Geometry: final body of the model. Coordinates: model frame, mm. Face numbers are marked on the shaded views. A direction names the side the tool comes from. Give positions to 0.01 mm unless a question says otherwise; leave off trailing zeros. Write each loop counter-clockwise with the first axis right and the second up, starting at its lowest first coordinate (ties: lowest second). Pieces come first, ordered by that corner, then holes. Notation, with made-up numbers: (-22, -0.75) -> (22, -0.75) arc R23 ccw to (22, 13.25) -> close; hole circle Ø9 at (16.25, -4.75). An arc over 180 degrees is marked (long way). Answer in a Markdown table with one row per item. Add a question column.
Item 1: Section query B-B on y = 51. Output: boundary loops of the cut face in (x, z) (3 decimals), plus the area to 3 significant figures.
Item 2: Section query A-A on z = -3.5. Output: boundary loops of the cut face in (x, y) (3 decimals).
Item 3: Draft query along X for the marked faces 4, 5, 6 and 7. Return one class per face: +X half, -X half, draft (parallel to the pull), parting line (faces both ways), or undercut.
Item 4: Access query for the marked faces 1, 2 and 3. Directions: +Z, -Z, +X, -X, +Y, -Y. A direction counts if a zero-diameter tool reaches every point of the face in a straight line with its end or side. Return the directions, or none.
Item 5: Material intervals for probe 1 along Z at (x, y) = (76, 20.5) (3 decimals); probe 2 along Z at (x, y) = (-21, -26) (3 decimals); probe 3 along X at (y, z) = (15.5, 8.5) (3 decimals), sorted ascending. Write a range as from..to.
Item 6: First-contact query: P1, Ø1, axis at y = 1, z = 15, coming from the -X side; P2, Ø15, axis at y = -25.5, z = 4, coming from the -X side (3 decimals); P3, Ø2.5, axis at y = -3, z = 40.5, coming from the -X side. Flat tips, straight axial feed; report the tip coordinate or a pass-through.
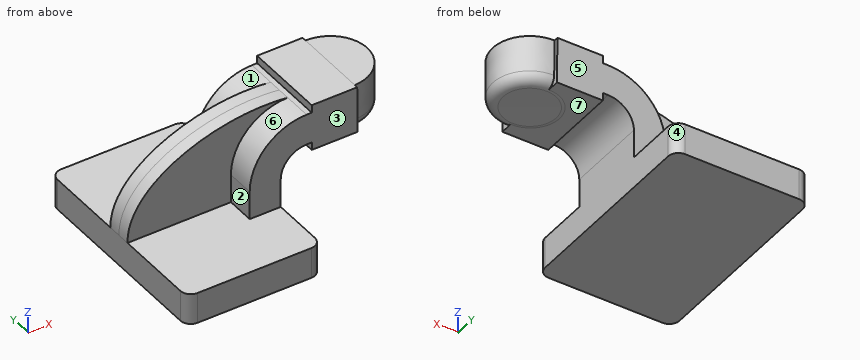
```python
from build123d import *

# Parameters (mm, degrees)
F1_DEPTH    = 63.5
F2_DEPTH    = 25.4
F3_DEPTH    = 7.9375
F5_T1_DEPTH = 50.8


# Not quite as in the source:
# - a fillet or chamfer that OpenCascade refuses, or shapes differently, is made with other operations: its cross-section is extruded or revolved along the edge and cut away or added


with BuildPart() as f1:
    # F0 (on Front) → F1 (new body, symmetric)
    with BuildSketch(Plane.XZ):
        Polygon((22.225, 9.525), (-41.275, 9.525), (-41.275, -9.525), (41.275, -9.525), (41.275, 9.525), align=None)
    extrude(amount=F1_DEPTH, both=True)

    # F0 (on Front) → F2 (join, symmetric)
    with BuildSketch(Plane.XZ):
        with BuildLine():
            Line((22.225, 27.0002), (22.225, 9.525))
            Line((22.225, 9.525), (41.275, 9.525))
            Line((41.275, 9.525), (41.275, 27.0002))
            ThreePointArc((41.275, 27.0002), (45.9246798487, 38.2255201513), (57.15, 42.8752))
            Line((57.15, 42.8752), (60.325, 42.8752))
            Line((60.325, 42.8752), (60.325, 61.9252))
            Line((60.325, 61.9252), (57.15, 61.9252))
            ThreePointArc((57.15, 61.9252), (32.4542956671, 51.6959043329), (22.225, 27.0002))
        make_face()
        Polygon((60.325, 66.675), (60.325, 61.9252), (60.325, 42.8752), (60.325, 38.1), (88.4848684072, 38.1), (88.2495848575, 66.675), align=None)
    extrude(amount=F2_DEPTH, both=True)

    # F0 (on Front) → F3 (join, symmetric)
    with BuildSketch(Plane.XZ):
        with BuildLine():
            add(Edge.make_bspline(
                [(-41.275, 9.525), (-41.8986715376, 44.9499189854), (12.7891246229, 67.7922144532), (57.15, 61.9252)],
                knots=[0, 0, 0, 0, 111.5045361635, 111.5045361635, 111.5045361635, 111.5045361635], degree=3))
            Line((-41.275, 9.525), (22.225, 9.525))
            Line((22.225, 9.525), (22.225, 27.0002))
            ThreePointArc((22.225, 27.0002), (32.4542956671, 51.6959043329), (57.15, 61.9252))
        make_face()
    extrude(amount=F3_DEPTH, both=True)

    # F0 (on Front) → F4 (revolve)
    with BuildSketch(Plane.XZ):
        Polygon((111.125, 66.675), (88.2495848575, 66.675), (88.4848684072, 38.1), (111.125, 38.1), align=None)
    revolve(axis=Axis((88.3672266324, 0, 52.3875), (-0.0082336159, 0, 0.9999661032)))

    # F5: fillet of radius 6.35 on 5 edges, made by hand

    # F5_s2 → F5_t1 (cut)
    with BuildSketch(Plane.XY.offset(-25.4)):
        with BuildLine():
            ThreePointArc((34.925, -63.5), (39.4151280605, -61.6401280605), (41.275, -57.15))
            Line((41.275, -57.15), (41.275, -63.5))
            Line((41.275, -63.5), (34.925, -63.5))
        make_face()
        with BuildLine():
            ThreePointArc((34.925, 63.5), (39.4151280605, 61.6401280605), (41.275, 57.15))
            Line((41.275, 57.15), (41.275, 63.5))
            Line((41.275, 63.5), (34.925, 63.5))
        make_face()
        with BuildLine():
            ThreePointArc((-34.925, 63.5), (-39.4151280605, 61.6401280605), (-41.275, 57.15))
            Line((-41.275, 57.15), (-41.275, 63.5))
            Line((-41.275, 63.5), (-34.925, 63.5))
        make_face()
        with BuildLine():
            ThreePointArc((-34.925, -63.5), (-39.4151280605, -61.6401280605), (-41.275, -57.15))
            Line((-41.275, -57.15), (-41.275, -63.5))
            Line((-41.275, -63.5), (-34.925, -63.5))
        make_face()
    extrude(amount=F5_T1_DEPTH, mode=Mode.SUBTRACT)


with BuildPart() as f5_tool4:
    # F5_s5 → F5_t6 (revolve)
    with BuildSketch(Plane.XZ):
        with BuildLine():
            ThreePointArc((111.125, 44.45), (109.2651280605, 39.9598719395), (104.775, 38.1))
            Line((104.775, 38.1), (111.125, 38.1))
            Line((111.125, 38.1), (111.125, 44.45))
        make_face()
    revolve(axis=Axis((88.4864032368, 0, 37.9135961712), (-0.0082336159, 0, 0.9999661032)))

    split(bisect_by=Plane(origin=(88.7925599353, 0, 0.7311086157), x_dir=(0, 1, 0), z_dir=(0.9999661032, 0, 0.0082336159)), keep=Keep.TOP)

    split(bisect_by=Plane.XY.offset(38.1), keep=Keep.TOP)


with BuildPart() as f1_1:
    add(f1.part)

    # F5_t3: cut F5_tool4
    add(f5_tool4.part, mode=Mode.SUBTRACT)


with BuildPart() as f5_tool10:
    # F5_s11 → F5_t12 (revolve)
    with BuildSketch(Plane.XZ):
        with BuildLine():
            ThreePointArc((111.125, 44.45), (109.2651280605, 39.9598719395), (104.775, 38.1))
            Line((104.775, 38.1), (111.125, 38.1))
            Line((111.125, 38.1), (111.125, 44.45))
        make_face()
    revolve(axis=Axis((88.4864032368, 0, 37.9135961712), (-0.0082336159, 0, 0.9999661032)))

    split(bisect_by=Plane(origin=(88.7925599353, 0, 0.7311086157), x_dir=(0, 1, 0), z_dir=(0.9999661032, 0, 0.0082336159)), keep=Keep.TOP)

    split(bisect_by=Plane.XY.offset(38.1), keep=Keep.BOTTOM)


with BuildPart() as f1_2:
    add(f1_1.part)

    # F5_t9: cut F5_tool10
    add(f5_tool10.part, mode=Mode.SUBTRACT)


with BuildPart() as f5_tool16:
    # F5_s17 → F5_t18 (revolve)
    with BuildSketch(Plane.XZ):
        with BuildLine():
            ThreePointArc((111.125, 44.45), (109.2651280605, 39.9598719395), (104.775, 38.1))
            Line((104.775, 38.1), (111.125, 38.1))
            Line((111.125, 38.1), (111.125, 44.45))
        make_face()
    revolve(axis=Axis((88.4864032368, 0, 37.9135961712), (-0.0082336159, 0, 0.9999661032)))

    split(bisect_by=Plane(origin=(88.7925599353, 0, 0.7311086157), x_dir=(0, 1, 0), z_dir=(-0.9999661032, 0, -0.0082336159)), keep=Keep.TOP)

    split(bisect_by=Plane.XY.offset(38.1), keep=Keep.BOTTOM)


with BuildPart() as f1_3:
    add(f1_2.part)

    # F5_t15: cut F5_tool16
    add(f5_tool16.part, mode=Mode.SUBTRACT)


solid = f1_3.part
```
Findings below:
| question | item | result |
|---|---|---|
| 1 | outline | (-41.275, -9.525) -> (41.275, -9.525) -> (41.275, 9.525) -> (-41.275, 9.525) -> close |
| 1 | area | 1,570 mm^2 |
| 2 | outline | (-41.275, -57.15) arc R6.35 ccw to (-34.925, -63.5) -> (34.925, -63.5) arc R6.35 ccw to (41.275, -57.15) -> (41.275, 57.15) arc R6.35 ccw to (34.925, 63.5) -> (-34.925, 63.5) arc R6.35 ccw to (-41.275, 57.15) -> close |
| 3 | face 4 | +X half |
| 3 | face 5 | draft |
| 3 | face 6 | -X half |
| 3 | face 7 | undercut |
| 4 | face 1 | +Z, -X, +Y |
| 4 | face 2 | +Z, -X, -Y |
| 4 | face 3 | +Z, +X, -X, -Y |
| 5 | probe 1 | z = 38.1..66.675 |
| 5 | probe 2 | z = -9.525..9.525 |
| 5 | probe 3 | x = -41.275..41.275 |
| 6 | P1 | stops at x = -40.99 |
| 6 | P2 | stops at x = -41.275 |
| 6 | P3 | stops at x = -26.91 |
